Could you check a few things on this drawing? It's one solid part, dimensions in mm from its lowest x, y, z. Give positions to 0.01 mm unless a question says otherwise; leave off trailing zeros. Order: outer loops, then holes, each group sorted by start corner. A loop starts at its lowest first (then second) coordinate and runs counter-clockwise, first axis right, second up.
(1) If I drill on probe 1 along Y at (x, z) = (3, 12); probe 2 along X at (y, z) = (4.5, 11.8); probe 3 along Z at (x, y) = (0.4, 5), over which ranges is the centre line in solid material (lowest first)?
(2) Imagine slicing it at A-A, the plane x = 1.1. Write out the boundary of the cut face in (y, z), then the cut area to 3 significant figures.
(3) Imagine slicing it at C-C, the plane z = 5. Write out the boundary of the cut face in (x, y), then the cut area to 3 significant figures.
(4) If we mould it in two halves opening along X, with no side actions, what happens to the marked faces 1, 2 and 3? For each: released by +X, released by -X, zero draft, split by the parting line, or undercut.
(5) Imagine slicing it at B-B, the plane z = 14.5. Write out the boundary of the cut face in (x, y).
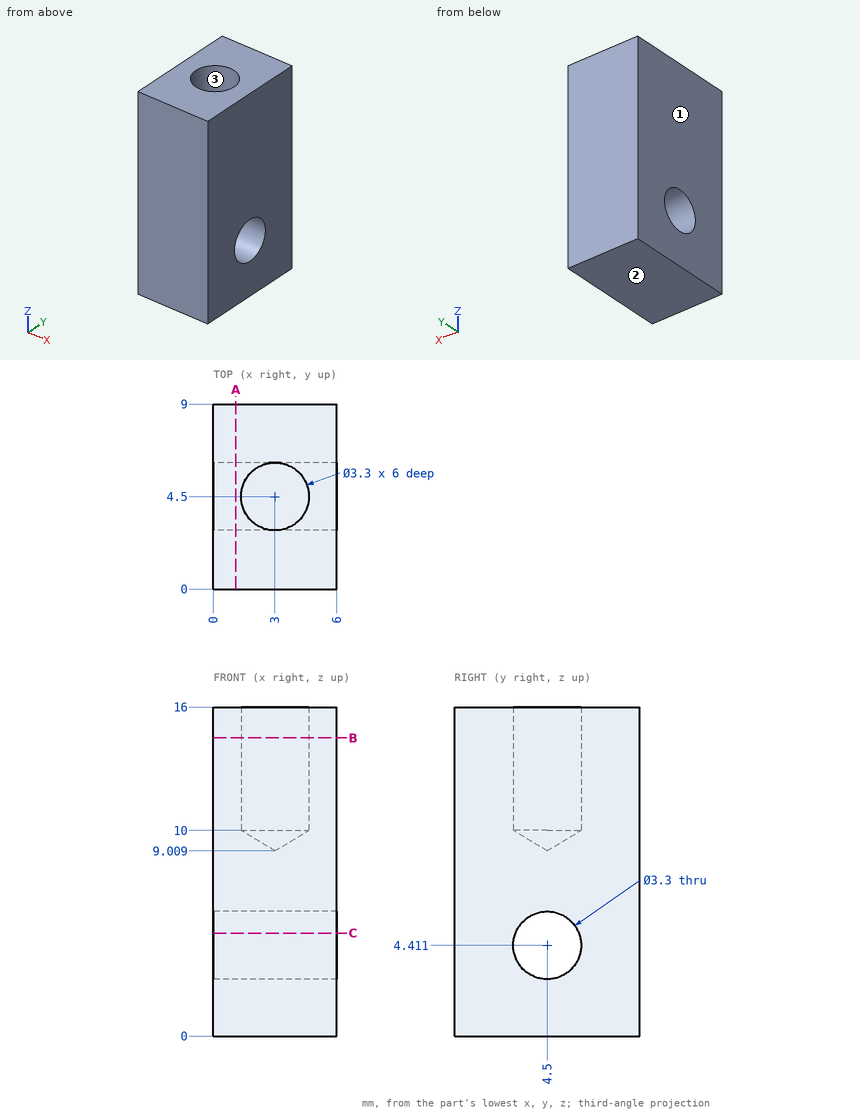
Answer block:
1. probe 1: y = 0 to 2.85, 6.15 to 9
1. probe 2: x = 0 to 1.35, 4.65 to 6
1. probe 3: z = 0 to 2.84, 5.98 to 16
2. outline: (0, 0) - (9, 0) - (9, 16) - (0, 16) - close; hole circle Ø3.3 at (4.5, 4.41)
2. area: 135 mm2
3. outline: (0, 0) - (6, 0) - (6, 2.96) - (0, 2.96) - close; (0, 6.04) - (6, 6.04) - (6, 9) - (0, 9) - close
3. area: 35.5 mm2
4. face 1: released by -X
4. face 2: zero draft
4. face 3: undercut
5. outline: (0, 0) - (6, 0) - (6, 9) - (0, 9) - close; hole circle Ø3.3 at (3, 4.5)
